Read the model definition and answer for the solid it produces. Units are mm, in the model's axes. A direction names the side the tool comes from. Give positions to 0.01 mm unless a question says otherwise; leave off trailing zeros. Write each loop counter-clockwise with the first axis right and the second up, starting at its lowest first coordinate (ties: lowest second). Pieces come first, ordered by that corner, then holes. Notation, with made-up numbers: (54, -35.5) -> (102, -35.5) arc R36 ccw to (102, -1.5) -> close; hole circle Ø3 at (37.5, -29.5). An arc over 180 degrees is marked (long way). Use a Markdown table: item, result.
from build123d import *

# Parameters (mm, degrees)
SKETCH1_W                      = 12.04
SKETCH1_H                      = 7.58
SKETCH1_W_2                    = 8.04
SKETCH1_H_2                    = 3.58
BOSS_EXTRUDE1_DEPTH            = 8
SKETCH1_2_W                    = 12.04
SKETCH1_2_H                    = 7.58
SKETCH1_2_W_2                  = 8.04
SKETCH1_2_H_2                  = 3.58
BOSS_EXTRUDE2_DEPTH            = 2
EXTRUDE_THIN1_DEPTH            = 12.04
SKETCH5_W                      = 12.04
SKETCH5_H                      = 7.58
SKETCH5_W_2                    = 8.04
SKETCH5_H_2                    = 3.58
BOSS_EXTRUDE4_DEPTH            = 8
SKETCH5_4_W                    = 12.04
SKETCH5_4_H                    = 7.58
BOSS_EXTRUDE5_DEPTH            = 2
CHAMFER1_SIZE                  = 1.5
CHAMFER2_START                 = -7
CHAMFER2_DEPTH                 = 14
CUT_EXTRUDE1_REACH             = 45.534
CUT_EXTRUDE1_DIRECTION_2_DEPTH = 44.534029429
CUT_EXTRUDE2_DEPTH             = 43.263143381
CUT_EXTRUDE2_DEPTH_BACK        = 43.263143381
SKETCH8_W                      = 2
SKETCH8_H                      = 1.58
CUT_EXTRUDE3_DEPTH             = 7
SKETCH9_W                      = 4
SKETCH9_H                      = 1.58
CUT_EXTRUDE4_DEPTH             = 7
BOSS_EXTRUDE7_DEPTH            = 0.3


with BuildPart() as part:
    # Sketch1 → Boss-Extrude1 (new body)
    with BuildSketch(Plane.XY):
        Rectangle(SKETCH1_W, SKETCH1_H)
        Rectangle(SKETCH1_W_2, SKETCH1_H_2, mode=Mode.SUBTRACT)
    extrude(amount=BOSS_EXTRUDE1_DEPTH)

    # Sketch1<2> → Boss-Extrude2 (add)
    # profile 1 of 2: a face of its own
    with BuildSketch(Plane.XY):
        Rectangle(SKETCH1_2_W, SKETCH1_2_H)
        Rectangle(SKETCH1_2_W_2, SKETCH1_2_H_2, mode=Mode.SUBTRACT)
    # profile 2 of 2: a face of its own
    with BuildSketch(Plane.XY):
        Rectangle(SKETCH1_2_W_2, SKETCH1_2_H_2)
    extrude(amount=-BOSS_EXTRUDE2_DEPTH)

    # Sketch3 → Extrude-Thin1 (add)
    with BuildSketch(Plane(origin=(6.02, 9.81, 0), x_dir=(0, -1, 0), z_dir=(1, 0, 0))):
        with BuildLine():
            Line((6.02, 2.744137986), (6.52, 2.744137986))
            ThreePointArc((6.52, 2.744137986), (10.07949931, 2.557592532), (13.6, 2))
            Line((13.6, 2), (21.425180806, 0.336706473))
            ThreePointArc((21.425180806, 0.336706473), (22.132801564, 0.448660765), (22.583941196, 1.005198215))
            ThreePointArc((22.583941196, 1.005198215), (25.714510404, 11.554301253), (28.285098031, 22.253652529))
            Line((28.285098031, 22.253652529), (28.472176136, 23.133785819))
            Line((28.472176136, 23.133785819), (30.428471338, 22.717962437))
            Line((30.428471338, 22.717962437), (30.241393232, 21.837829148))
            ThreePointArc((30.241393232, 21.837829148), (27.646188069, 11.036014268), (24.485638594, 0.385886497))
            ThreePointArc((24.485638594, 0.385886497), (23.132219698, -1.283725852), (21.009357424, -1.619588728))
            Line((21.009357424, -1.619588728), (13.184176618, 0.043704799))
            ThreePointArc((13.184176618, 0.043704799), (9.870442383, 0.568548741), (6.52, 0.744137986))
            Line((6.52, 0.744137986), (6.02, 0.744137986))
            Line((6.02, 0.744137986), (6.02, 2.744137986))
        make_face()
    extrude(amount=-EXTRUDE_THIN1_DEPTH)



with BuildPart() as body_2:
    # Sketch5 → Boss-Extrude4 (new body)
    with BuildSketch(Plane(origin=(0, 485.418561105, -130.279454131), x_dir=(1, 0, 0), z_dir=(0, -0.20791169081775487, -0.9781476007338067))):
        with Locations((0, 517.132200771)):
            Rectangle(SKETCH5_W, SKETCH5_H)
        with Locations((0, 517.132200771)):
            Rectangle(SKETCH5_W_2, SKETCH5_H_2, mode=Mode.SUBTRACT)
    extrude(amount=BOSS_EXTRUDE4_DEPTH)


with BuildPart() as part_1:
    add(part.part)

    add(body_2.part)  # Boss-Extrude5 merges body 2
    # Sketch5<4> → Boss-Extrude5 (add)
    with BuildSketch(Plane(origin=(0, 485.418561105, -130.279454131), x_dir=(1, 0, 0), z_dir=(0, -0.20791169081775487, -0.9781476007338067))):
        with Locations((0, 517.132200771)):
            Rectangle(SKETCH5_4_W, SKETCH5_4_H)
    extrude(amount=-BOSS_EXTRUDE5_DEPTH)

    # Chamfer1
    chamfer1_edges = [part_1.edges().sort_by_distance(p)[0] for p in [
        (6.02, -24.743974821, -24.908081386),
        (-6.02, -24.743974821, -24.908081386),
        (6.02, 3.79, 2.627931007),
        (6.02, -3.79, 4.022340595),
        (-6.02, -3.79, 4.022340595),
        (-6.02, 3.79, 2.627931007),
        (6.02, -17.329616007, -26.484052003),
        (-6.02, -17.329616007, -26.484052003),
    ]]
    chamfer(chamfer1_edges, length=CHAMFER1_SIZE)

    # Chamfer2: read off the stored shape, not the designer's step
    # Chamfer2 outline → Chamfer2 (cut)
    with BuildSketch(Plane.YZ.offset(CHAMFER2_START)):
        with BuildLine():
            Line((3.79, -2.744137986), (3.79, -0.709020541))
            Line((3.79, -0.709020541), (1.696404781, -2.706829325))
            ThreePointArc((1.696404781, -2.706829325), (2.492984056, -2.734809543), (3.29, -2.744137986))
            Line((3.29, -2.744137986), (3.79, -2.744137986))
        make_face()
        Polygon((-23.704416367, -20.017343383), (-24.120239749, -21.973638584), (-21.748121165, -20.433166764), align=None)
        with BuildLine():
            ThreePointArc((-18.243518062, -21.17809315), (-18.243825174, -21.1795015), (-18.244132277, -21.180909853))
            Line((-18.244132277, -21.180909853), (-16.705880935, -23.549609201))
            Line((-16.705880935, -23.549609201), (-16.290057553, -21.593313999))
            Line((-16.290057553, -21.593313999), (-18.243518062, -21.17809315))
        make_face()
    extrude(amount=CHAMFER2_DEPTH, mode=Mode.SUBTRACT)

    # Cut-Extrude1: up to this face of the body (flat: up to its plane)
    cut_extrude1_end = Plane(part_1.part.faces().sort_by_distance((0, -3.79, 4.022340595))[0])
    # Sketch6 → Cut-Extrude1 (cut, up to the picked face)
    with BuildSketch(Plane(origin=(0, 3.79, 0), x_dir=(1, 0, 0), z_dir=(0, 1, 0)), mode=Mode.PRIVATE) as cut_extrude1_sk1:
        with BuildLine():
            Line((1.45, -3.566987298), (-0.35, -2.527756814))
            ThreePointArc((-0.35, -2.527756814), (-0.85, -2.527756814), (-1.1, -2.960769515))
            Line((-1.1, -2.960769515), (-1.1, -5.039230485))
            ThreePointArc((-1.1, -5.039230485), (-0.85, -5.472243186), (-0.35, -5.472243186))
            Line((-0.35, -5.472243186), (1.45, -4.433012702))
            ThreePointArc((1.45, -4.433012702), (1.7, -4), (1.45, -3.566987298))
        make_face()
    cut_extrude1_tool1 = split(extrude(cut_extrude1_sk1.sketch, amount=-CUT_EXTRUDE1_REACH, mode=Mode.PRIVATE), bisect_by=cut_extrude1_end, keep=Keep.BOTH, mode=Mode.PRIVATE)
    add(cut_extrude1_tool1.solids().sort_by(Axis((0, 3.79, 4), (0, -1, 0)))[0], mode=Mode.SUBTRACT)

    # Sketch6 → Cut-Extrude1 direction 2 (cut)
    with BuildSketch(Plane(origin=(0, 3.79, 0), x_dir=(1, 0, 0), z_dir=(0, 1, 0))):
        with BuildLine():
            Line((1.45, -3.566987298), (-0.35, -2.527756814))
            ThreePointArc((-0.35, -2.527756814), (-0.85, -2.527756814), (-1.1, -2.960769515))
            Line((-1.1, -2.960769515), (-1.1, -5.039230485))
            ThreePointArc((-1.1, -5.039230485), (-0.85, -5.472243186), (-0.35, -5.472243186))
            Line((-0.35, -5.472243186), (1.45, -4.433012702))
            ThreePointArc((1.45, -4.433012702), (1.7, -4), (1.45, -3.566987298))
        make_face()
    extrude(amount=CUT_EXTRUDE1_DIRECTION_2_DEPTH, mode=Mode.SUBTRACT)

    # Sketch7 → Cut-Extrude2 (cut, two sides: drawn at the far end of the back side and taken through both)
    with BuildSketch(Plane(origin=(0, -18.608845607, 3.955432239), x_dir=(1, 0, 0), z_dir=(0, -0.9781476007338067, 0.2079116908177549)).offset(-CUT_EXTRUDE2_DEPTH_BACK)):
        with BuildLine():
            Line((1.45, -30.075328988), (-0.35, -29.036098503))
            ThreePointArc((-0.35, -29.036098503), (-0.85, -29.036098503), (-1.1, -29.469111205))
            Line((-1.1, -29.469111205), (-1.1, -31.547572174))
            ThreePointArc((-1.1, -31.547572174), (-0.85, -31.980584876), (-0.35, -31.980584876))
            Line((-0.35, -31.980584876), (1.45, -30.941354391))
            ThreePointArc((1.45, -30.941354391), (1.7, -30.508341689), (1.45, -30.075328988))
        make_face()
    extrude(amount=CUT_EXTRUDE2_DEPTH + CUT_EXTRUDE2_DEPTH_BACK, mode=Mode.SUBTRACT)

    # Sketch8 → Cut-Extrude3 (cut)
    with BuildSketch(Plane.XY.offset(8)):
        with Locations((5.02, 0)):
            Rectangle(SKETCH8_W, SKETCH8_H)
    extrude(amount=-CUT_EXTRUDE3_DEPTH, mode=Mode.SUBTRACT)

    # Sketch9 → Cut-Extrude4 (cut)
    with BuildSketch(Plane(origin=(0, -7.174687668, -33.754251629), x_dir=(-1, 0, 0), z_dir=(0, -0.20791169081775673, -0.9781476007338064))):
        with Locations((-6.02, -15.234578288)):
            Rectangle(SKETCH9_W, SKETCH9_H)
    extrude(amount=-CUT_EXTRUDE4_DEPTH, mode=Mode.SUBTRACT)

    # Sketch11 → Boss-Extrude7 (add)
    with BuildSketch(Plane(origin=(6.02, 0, -6.02), x_dir=(0, 0, 1), z_dir=(-1, 0, 0))):
        with BuildLine():
            Line((5.047536003, 0.082682927), (5.047536003, 0.79))
            Line((5.047536003, 0.79), (4.608511613, 0.79))
            Line((4.608511613, 0.79), (4.608511613, -1.21))
            Line((4.608511613, -1.21), (5.299060394, -1.21))
            add(Edge.make_bspline(
                [(5.299060394, -1.21), (5.329313952, -1.209669089), (5.387892505, -1.20902836), (5.472763934, -1.201041655), (5.551912875, -1.189213366), (5.625349672, -1.172100798), (5.693083305, -1.150229064), (5.754766894, -1.122952683), (5.811034602, -1.091546463), (5.860787755, -1.054159212), (5.905113914, -1.0123961), (5.943543862, -0.965606031), (5.975708858, -0.913602215), (6.002058422, -0.856769543), (6.02273613, -0.795055664), (6.036919265, -0.728309994), (6.045834622, -0.656886984), (6.046958484, -0.607639268), (6.047536003, -0.582332317)],
                knots=[0, 0, 0, 0, 1.298309684, 2.513856393, 3.656108695, 4.731525363, 5.747269452, 6.706842141, 7.622696522, 8.50723259, 9.371308978, 10.231556582, 11.09863924, 11.989139744, 12.915198226, 13.88644584, 14.913906774, 16, 16, 16, 16], degree=3))
            add(Edge.make_bspline(
                [(6.047536003, -0.582332317), (6.046958026, -0.557515305), (6.045826057, -0.50891113), (6.034579341, -0.43810911), (6.01784318, -0.370657155), (5.992755465, -0.307388849), (5.96129274, -0.247554648), (5.922654871, -0.191755979), (5.876715772, -0.140008785), (5.824737087, -0.092263463), (5.76741001, -0.049357043), (5.705904977, -0.012393475), (5.640949178, 0.01871881), (5.572580865, 0.043912433), (5.500609023, 0.062967718), (5.425113901, 0.075859677), (5.346196751, 0.08276557), (5.2924674, 0.082710787), (5.265142711, 0.082682927)],
                knots=[0, 0, 0, 0, 1.030031435, 2.017318961, 2.9707634, 3.911434012, 4.836705747, 5.773461207, 6.723043161, 7.705184701, 8.700351159, 9.692154612, 10.681034209, 11.68770297, 12.714187277, 13.76904456, 14.865421547, 16, 16, 16, 16], degree=3))
            Line((5.265142711, 0.082682927), (5.047536003, 0.082682927))
        make_face()
        with BuildLine():
            Line((5.036103077, -0.892926829), (5.036103077, -0.234390244))
            Line((5.036103077, -0.234390244), (5.224746369, -0.234390244))
            add(Edge.make_bspline(
                [(5.224746369, -0.234390244), (5.240257069, -0.234519065), (5.270324289, -0.234768783), (5.313827436, -0.239266362), (5.354507641, -0.245501395), (5.39208054, -0.254654559), (5.426930993, -0.265974439), (5.458434732, -0.280437451), (5.487059955, -0.297407138), (5.512929634, -0.316804387), (5.535224382, -0.339455254), (5.555117628, -0.364216963), (5.571992729, -0.391655317), (5.585050634, -0.422099729), (5.596087863, -0.45462628), (5.602917978, -0.490012993), (5.607750907, -0.527828853), (5.608252881, -0.553986887), (5.608511613, -0.567469512)],
                knots=[0, 0, 0, 0, 1.278264899, 2.477894098, 3.602370215, 4.669373304, 5.663063542, 6.619223296, 7.520996807, 8.402964925, 9.276935434, 10.134111266, 11.017943356, 11.922995833, 12.86038281, 13.844364746, 14.88892179, 16, 16, 16, 16], degree=3))
            add(Edge.make_bspline(
                [(5.608511613, -0.567469512), (5.608243066, -0.580569264), (5.607719879, -0.606090356), (5.602979451, -0.643045607), (5.595872643, -0.677668866), (5.585733194, -0.709706236), (5.572188175, -0.739091862), (5.555687516, -0.765952955), (5.536368124, -0.790420284), (5.513666923, -0.811964985), (5.488692805, -0.831640584), (5.459986472, -0.847894241), (5.428669687, -0.862115985), (5.394268426, -0.873426519), (5.357002183, -0.882096268), (5.316907649, -0.888585203), (5.273728574, -0.892402235), (5.243936115, -0.892748228), (5.228557345, -0.892926829)],
                knots=[0, 0, 0, 0, 1.096807385, 2.136813243, 3.115574441, 4.054422268, 4.94474187, 5.818891163, 6.689666352, 7.547538513, 8.435055958, 9.345744162, 10.302983784, 11.312439221, 12.373194966, 13.505006157, 14.712092391, 16, 16, 16, 16], degree=3))
            Line((5.228557345, -0.892926829), (5.036103077, -0.892926829))
        make_face(mode=Mode.SUBTRACT)
    extrude(amount=-BOSS_EXTRUDE7_DEPTH)


solid = part_1.part
Item 1: Straight lines are drawn through the part: line 1 along Y through (x, z) = (-1.75, 6); line 2 along X through (y, z) = (-6.5, 0.5); line 3 along Y through (x, z) = (-2.25, -24). For each, find the intervals that lie inside material, in ascending order. Write a range as [from, to].
Return value:
| item | result |
|---|---|
| line 1 | [-3.79, -1.79], [1.79, 3.79] |
| line 2 | [-6.02, 6.02] |
| line 3 | [-24.55, -22.51], [-18.85, -16.8] |
Item 2: Each of these flat-tipped pins is pushed along its axis until it touches: P1, Ø1.8, axis at y = -0.5, z = 5, coming from the +X side; P2, Ø1.8, axis at x = 1, y = -0.5, coming from the +Z side; P3, Ø1.5, axis at x = -1.5, z = -21.5, coming from the +Y side; P4, Ø1.5, axis at y = -0.5, z = -4, coming from the -X side. Where does it stop, or does it pass through?
Return value:
| item | result |
|---|---|
| P1 | x = 6.02 |
| P2 | z = 0 |
| P3 | y = -17.55 |
| P4 | through |
Item 3: A cutting plane is placed at B-B (z = -6). Give the vertices of the cut face in (x, y), then the cut area to 3 significant figures.
Return value:
| item | result |
|---|---|
| outline | (-6.02, -16.42) -> (6.02, -16.42) -> (6.02, -14.33) -> (-6.02, -14.33) -> close |
| area | 25.1 mm^2 |
Item 4: A cutting plane is placed at C-C (y = -15.5). Give the vertices of the cut face in (x, z).
Return value:
| item | result |
|---|---|
| outline | (-6.02, -10.07) -> (6.02, -10.07) -> (6.02, -2.97) -> (-6.02, -2.97) -> close |
Item 5: For a pull along Y with two mould halves and no side action, classify faces 1 (the face through (0.537, -24.16, -27.036)), 2 (the face through (0.084, -6.807, 0.686)), 3 (the face through (0.563, -2.776, 3.055)), 4 (the face through (-5.259, -24.086, -25.371)) as +Y half, -Y half, draft (parallel to the pull), parting line (faces both ways), or undercut.
Return value:
| item | result |
|---|---|
| face 1 | undercut |
| face 2 | undercut |
| face 3 | draft |
| face 4 | -Y half |
Item 6: A tool of negligible diameter and unlimited length cuts with its end or side. For faces 5 (the face through (-1.1, -3, 4)), 6 (the face through (-4.02, 0, 4)), 7 (the face through (4.02, -20, -27)), 8 (the face through (0.56, -23.76, -25.17)), 9 (the face through (-0.86, -24.27, -27.53)), from which of +Z, -Z, +X, -X, +Y, -Y can it reach the whole face along a straight path? Write none if from no direction.
Return value:
| item | result |
|---|---|
| face 5 | +Y, -Y |
| face 6 | +Z |
| face 7 | none |
| face 8 | -Y |
| face 9 | +Y |
